Read the model definition and answer for the solid it produces. Units are mm, in the model's axes. A direction names the side the tool comes from. Round coordinates to 2 decimals unless told otherwise and drop trailing zeros. Loops run counter-clockwise (first coordinate to the right, second up) from the corner with the lowest first, then second, coordinate; pieces in that order, holes last. Notation, with made-up numbers: (39.25, -23) - (43.25, -23) arc R21 cw to (43.25, 0) - close; hole circle Ø2 at (88, 47.5). An arc over 180 degrees is marked (long way). Answer as CSV lines item,"result".
```python
from build123d import *

# Parameters (mm, degrees)
EXTRUDE_1_DEPTH      = 2
EXTRUDE_2_DEPTH      = 4
EXTRUDE_2_DEPTH_BACK = 5
SKETCH_3_R           = 5
CUT_EXTRUDE_1_DEPTH  = 2
SKETCH_4_R           = 1.5
CUT_EXTRUDE_2_DEPTH  = 2
SKETCH_5_R           = 3
CUT_EXTRUDE_3_DEPTH  = 5
EXTRUDE_3_REACH      = 51.588
CHAMFER_1_SIZE       = 0.2
CHAMFER_2_SIZE       = 0.2
CHAMFER_3_SIZE       = 0.2
CHAMFER_4_ANGLE      = 180
CHAMFER_5_SIZE       = 0.2


with BuildPart() as part:
    # 草图1 → 凸台-拉伸1 (new body)
    with BuildSketch(Plane(origin=(0, 0, 0), x_dir=(0, 0, -1), z_dir=(1, 0, 0))):
        with BuildLine():
            ThreePointArc((-4, 0), (-2.828427125, -2.828427125), (0, -4))
            Line((0, -4), (0, -1.5))
            ThreePointArc((0, -1.5), (-1.5, 0), (0, 1.5))
            Line((0, 1.5), (0, 3.5))
            ThreePointArc((0, 3.5), (-1.5, 5), (0, 6.5))
            Line((0, 6.5), (0, 8.5))
            ThreePointArc((0, 8.5), (-1.5, 10), (0, 11.5))
            Line((0, 11.5), (0, 13.5))
            ThreePointArc((0, 13.5), (-1.5, 15), (0, 16.5))
            Line((0, 16.5), (0, 18.5))
            ThreePointArc((0, 18.5), (-1.5, 20), (0, 21.5))
            Line((0, 21.5), (0, 31))
            ThreePointArc((0, 31), (-4.794759251, 32.596072789), (-7.67632231, 36.747429069))
            ThreePointArc((-7.67632231, 36.747429069), (-4.127055678, 18.544898625), (-4, 0))
        make_face()
        with BuildLine():
            Line((0, -1.5), (0, -4))
            ThreePointArc((0, -4), (2.828427125, -2.828427125), (4, 0))
            ThreePointArc((4, 0), (4.127055678, 18.544898625), (7.67632231, 36.747429069))
            ThreePointArc((7.67632231, 36.747429069), (4.794759251, 32.596072789), (0, 31))
            Line((0, 31), (0, 21.5))
            ThreePointArc((0, 21.5), (1.060660172, 21.060660172), (1.5, 20))
            ThreePointArc((1.5, 20), (1.060660172, 18.939339828), (0, 18.5))
            Line((0, 18.5), (0, 16.5))
            ThreePointArc((0, 16.5), (1.060660172, 16.060660172), (1.5, 15))
            ThreePointArc((1.5, 15), (1.060660172, 13.939339828), (0, 13.5))
            Line((0, 13.5), (0, 11.5))
            ThreePointArc((0, 11.5), (1.060660172, 11.060660172), (1.5, 10))
            ThreePointArc((1.5, 10), (1.060660172, 8.939339828), (0, 8.5))
            Line((0, 8.5), (0, 6.5))
            ThreePointArc((0, 6.5), (1.060660172, 6.060660172), (1.5, 5))
            ThreePointArc((1.5, 5), (1.060660172, 3.939339828), (0, 3.5))
            Line((0, 3.5), (0, 1.5))
            ThreePointArc((0, 1.5), (1.060660172, 1.060660172), (1.5, 0))
            ThreePointArc((1.5, 0), (1.060660172, -1.060660172), (0, -1.5))
        make_face()
    extrude(amount=EXTRUDE_1_DEPTH)

    # 草图2 → 凸台-拉伸2 (add, two sides: drawn at the far end of the back side and taken through both)
    with BuildSketch(Plane(origin=(0, 0, 0), x_dir=(0, 0, -1), z_dir=(1, 0, 0)).offset(-EXTRUDE_2_DEPTH_BACK)):
        with BuildLine():
            ThreePointArc((0, 47), (-8, 39), (0, 31))
            Line((0, 31), (0, 47))
        make_face()
        with BuildLine():
            Line((0, 47), (0, 31))
            ThreePointArc((0, 31), (5.656854249, 33.343145751), (8, 39))
            ThreePointArc((8, 39), (5.656854249, 44.656854249), (0, 47))
        make_face()
    extrude(amount=EXTRUDE_2_DEPTH + EXTRUDE_2_DEPTH_BACK)

    # 草图3 → 切除-拉伸1 (cut)
    with BuildSketch(Plane(origin=(4, 0, 0), x_dir=(0, 0, -1), z_dir=(1, 0, 0))):
        with Locations((0, 39)):
            Circle(SKETCH_3_R)
    extrude(amount=-CUT_EXTRUDE_1_DEPTH, mode=Mode.SUBTRACT)

    # 草图4 → 切除-拉伸2 (cut)
    with BuildSketch(Plane(origin=(2, 0, 0), x_dir=(0, 0, -1), z_dir=(1, 0, 0))):
        with Locations((0, 39)):
            Circle(SKETCH_4_R)
    extrude(amount=-CUT_EXTRUDE_2_DEPTH, mode=Mode.SUBTRACT)

    # 草图5 → 切除-拉伸3 (cut)
    with BuildSketch(Plane.ZY.offset(5)):
        with Locations((0, 39)):
            Circle(SKETCH_5_R)
    extrude(amount=-CUT_EXTRUDE_3_DEPTH, mode=Mode.SUBTRACT)

    # 草图7 → 凸台-拉伸3 (add, up to next)
    with BuildSketch(Plane.XY.offset(7), mode=Mode.PRIVATE) as extrude_3_sk1:
        with BuildLine():
            Line((-4.005881134, 42.683822956), (-0.994118866, 42.683822956))
            ThreePointArc((-0.994118866, 42.683822956), (-2.5, 46), (-4.005881134, 42.683822956))
        make_face()
    extrude_3_tool1 = extrude(extrude_3_sk1.sketch, amount=-EXTRUDE_3_REACH, mode=Mode.PRIVATE) - part.part
    add(extrude_3_tool1.solids().sort_by_distance((-2.5, 44.204391, 7))[0])

    # 倒角1
    chamfer_1_edges = [part.edges().sort_by_distance(p)[0] for p in [
        (-5, 39, -3),
        (4, 31, 0),
        (-5, 31, 0),
        (-2.5, 46, 7),
        (4, 39, 5),
    ]]
    chamfer(chamfer_1_edges, length=CHAMFER_1_SIZE)

    # 倒角2
    chamfer_2_edges = [part.edges().sort_by_distance(p)[0] for p in [
        (2, 1.5, 0),
        (0, 21.5, 0),
        (0, 16.5, 0),
        (0, 11.5, 0),
        (2, 6.5, 0),
        (0, 6.5, 0),
        (0, 1.5, 0),
        (2, 11.5, 0),
        (2, 16.5, 0),
        (2, 21.5, 0),
    ]]
    chamfer(chamfer_2_edges, length=CHAMFER_2_SIZE)

    # 倒角3
    # the kernel refuses this chamfer: 0.2 mm, written as the material it takes off along each edge
    with BuildSketch(Plane(origin=(0, 8.590292429, 103.630351179), x_dir=(0, 0.3061524264248754, -0.9519825060336777), z_dir=(0, 0.9519825060336777, 0.3061524264248754))) as chamfer_3_piece_1_section:
        Polygon((100 + CHAMFER_3_SIZE, 0), (100, -CHAMFER_3_SIZE), (100, 0), align=None)
    chamfer_3_piece_1 = revolve(axis=Axis((0, 8.590292429, 103.630351179), (-1, 0, 0)), revolution_arc=23.639557958, mode=Mode.PRIVATE)
    chamfer_3_piece_1 = chamfer_3_piece_1 - Plane(origin=(0, 39, 0), x_dir=(0, 1, 0), z_dir=(-1, 0, 0)) * Cylinder(8, 401, mode=Mode.PRIVATE)
    add(chamfer_3_piece_1, mode=Mode.SUBTRACT)
    with BuildSketch(Plane(origin=(0, 8.590292429, -103.630351179), x_dir=(0, -0.10126549371899889, 0.9948594371979629), z_dir=(0, -0.9948594371979629, -0.10126549371899889))) as chamfer_3_piece_2_section:
        Polygon((100 + CHAMFER_3_SIZE, 0), (100, -CHAMFER_3_SIZE), (100, 0), align=None)
    chamfer_3_piece_2 = revolve(axis=Axis((0, 8.590292429, -103.630351179), (-1, 0, 0)), revolution_arc=23.639557958, mode=Mode.PRIVATE)
    chamfer_3_piece_2 = chamfer_3_piece_2 - Plane(origin=(0, 39, 0), x_dir=(0, 1, 0), z_dir=(-1, 0, 0)) * Cylinder(8, 401, mode=Mode.PRIVATE)
    add(chamfer_3_piece_2, mode=Mode.SUBTRACT)
    with BuildSketch(Plane(origin=(2, 8.590292429, -103.630351179), x_dir=(0, -0.10126549371899889, 0.9948594371979629), z_dir=(0, -0.9948594371979629, -0.10126549371899889))) as chamfer_3_piece_3_section:
        Polygon((100, CHAMFER_3_SIZE), (100 + CHAMFER_3_SIZE, 0), (100, 0), align=None)
    chamfer_3_piece_3 = revolve(axis=Axis((2, 8.590292429, -103.630351179), (-1, 0, 0)), revolution_arc=23.639557958, mode=Mode.PRIVATE)
    chamfer_3_piece_3 = chamfer_3_piece_3 - Plane(origin=(2, 39, 0), x_dir=(0, 1, 0), z_dir=(-1, 0, 0)) * Cylinder(8, 401, mode=Mode.PRIVATE)
    add(chamfer_3_piece_3, mode=Mode.SUBTRACT)
    with BuildSketch(Plane(origin=(2, 8.590292429, 103.630351179), x_dir=(0, 0.3061524264248754, -0.9519825060336777), z_dir=(0, 0.9519825060336777, 0.3061524264248754))) as chamfer_3_piece_4_section:
        Polygon((100, CHAMFER_3_SIZE), (100 + CHAMFER_3_SIZE, 0), (100, 0), align=None)
    chamfer_3_piece_4 = revolve(axis=Axis((2, 8.590292429, 103.630351179), (-1, 0, 0)), revolution_arc=23.639557958, mode=Mode.PRIVATE)
    chamfer_3_piece_4 = chamfer_3_piece_4 - Plane(origin=(2, 39, 0), x_dir=(0, 1, 0), z_dir=(-1, 0, 0)) * Cylinder(8, 401, mode=Mode.PRIVATE)
    add(chamfer_3_piece_4, mode=Mode.SUBTRACT)

    # 倒角4: read off the stored shape, not the designer's step
    # 倒角4 outline → 倒角4 (revolve, cut)
    with BuildSketch(Plane.ZX):
        Polygon((4, 2), (3.8, 2), (4, 1.8), align=None)
        Polygon((4, 0), (4, 0.2), (3.8, 0), align=None)
    revolve(axis=Axis((0, 0, 0), (1, 0, 0)), revolution_arc=CHAMFER_4_ANGLE, mode=Mode.SUBTRACT)

    # 倒角5
    chamfer_5_edges = [part.edges().sort_by_distance(p)[0] for p in [
        (2, 39, 1.5),
    ]]
    chamfer(chamfer_5_edges, length=CHAMFER_5_SIZE)


solid = part.part
```
1) Find the intervals of material crossed by line 1 (Y direction, x = -4.25, z = 0); line 2 (Y direction, x = 2.65, z = 0); line 3 (X direction, y = 28.5, z = 1.5), in increasing order.
Entries:
line 1,"y = 31 to 36, 42 to 47"
line 2,"y = 31 to 34, 44 to 47"
line 3,"x = 0 to 2"
2) A cutting plane is placed at B-B, the plane z = -0.5. Count the separate pieces of the cut face and the enclosed holes in it, plus the area to 3 significant figures.
Entries:
separate pieces,"7"
enclosed holes,"0"
area,"130 mm^2"
3) Each of these flat-tipped pins is pushed along its axis until it touches: P1, Ø3, axis at x = -3, z = 3.5, coming from the +Y side; P2, Ø3, axis at x = -4, z = 2, coming from the +Y side; P3, Ø5, axis at y = 39, z = 0, coming from the -X side. Where does it stop, or does it pass through?
Entries:
P1,"stops at y = 46.75"
P2,"stops at y = 46.98"
P3,"stops at x = 0"
4) The mould has two halves that part along Y. Classify faces 1 (the face through (0, 16, 2)), 2 (the face through (0.989, 18.804, 4.153)): pulls with the +Y half, pulls with the -Y half, needs draft (parallel to the pull), parting line crosses it, or undercut.
Entries:
face 1,"needs draft"
face 2,"undercut"
5) A cutting plane is placed at A-A, the plane x = -2.5. Determine the outline of the cut face in (y, z), plus the area to 3 significant figures.
Entries:
outline,"(42.87, 7) arc R8 ccw (long way) to (46, 3.87) - (46, 6.8) - (45.8, 7) - close; hole circle Ø6 at (39, 0)"
area,"177 mm^2"
6) A tool of negligible diameter and unlimited length cuts with its end or side. For faces 3 (the face through (2.913, 43.957, 0.651)), 4 (the face through (0.99, 18.29, -4.1)), 5 (the face through (0, 37.7, 1.3)), 6 (the face through (-3, 44, 7)), 7 (the face through (0.913, 37.536, 0.325)), from which of +Z, -Z, +X, -X, +Y, -Y can it reach the whole face along a straight path? Write none if from no direction.
Entries:
face 3,"+X"
face 4,"-Z, +X, -X"
face 5,"-X"
face 6,"+Z, +X, -X, +Y"
face 7,"+X, -X"
